Autodesk Inventor part; units mm, degrees
ref_plane "YZ Plane" through (0, 0, 0) normal (1, 0, 0) x (0, 1, 0)
ref_plane "XZ Plane" through (0, 0, 0) normal (0, 1, 0) x (-1, 0, 0)
ref_plane "XY Plane" through (0, 0, 0) normal (0, 0, 1) x (1, 0, 0)
sketch "Sketch2" plane through (0, 0, 0) normal (0, 1, 0) x (-1, 0, 0)
  line L0 (-100, 22.5) -> (100, 22.5)
  line L1 (100, 22.5) -> (100, -22.5)
  line L2 (100, -22.5) -> (-100, -22.5)
  line L3 (-100, -22.5) -> (-100, 22.5)
  line L4 (-100, 22.5) -> (100, -22.5) construction
  line L5 (100, 22.5) -> (-100, -22.5) construction
  line L6 (100, 22.5) -> (95, 22.5)
  line L7 (95, 22.5) -> (95, 27.5)
  line L8 (95, 27.5) -> (100, 27.5)
  line L9 (100, 27.5) -> (100, 22.5)
  line L10 (100, -22.5) -> (95, -22.5)
  line L11 (95, -22.5) -> (95, -27.5)
  line L12 (95, -27.5) -> (100, -27.5)
  line L13 (100, -27.5) -> (100, -22.5)
  line L14 (-100, -22.5) -> (-90, -22.5)
  line L15 (-90, -22.5) -> (-90, -27.5)
  line L16 (-90, -27.5) -> (-100, -27.5)
  line L17 (-100, -27.5) -> (-100, -22.5)
  line L18 (-100, 22.5) -> (-90, 22.5)
  line L19 (-90, 22.5) -> (-90, 27.5)
  line L20 (-90, 27.5) -> (-100, 27.5)
  line L21 (-100, 27.5) -> (-100, 22.5)
  line L22 (94, 17.5) -> (82, 17.5)
  line L23 (82, 17.5) -> (82, 11.5)
  line L24 (82, 11.5) -> (94, 11.5)
  line L25 (94, 11.5) -> (94, 17.5)
  line L26 (70, 17.5) -> (58, 17.5)
  line L27 (70, 11.5) -> (70, 17.5)
  line L28 (58, 11.5) -> (70, 11.5)
  line L29 (58, 17.5) -> (58, 11.5)
  line L30 (46, 17.5) -> (34, 17.5)
  line L31 (46, 11.5) -> (46, 17.5)
  line L32 (34, 11.5) -> (46, 11.5)
  line L33 (34, 17.5) -> (34, 11.5)
  line L34 (22, 17.5) -> (10, 17.5)
  line L35 (22, 11.5) -> (22, 17.5)
  line L36 (10, 11.5) -> (22, 11.5)
  line L37 (10, 17.5) -> (10, 11.5)
  line L38 (-2, 17.5) -> (-14, 17.5)
  line L39 (-2, 11.5) -> (-2, 17.5)
  line L40 (-14, 11.5) -> (-2, 11.5)
  line L41 (-14, 17.5) -> (-14, 11.5)
  line L42 (-26, 17.5) -> (-38, 17.5)
  line L43 (-26, 11.5) -> (-26, 17.5)
  line L44 (-38, 11.5) -> (-26, 11.5)
  line L45 (-38, 17.5) -> (-38, 11.5)
  line L46 (-50, 17.5) -> (-62, 17.5)
  line L47 (-50, 11.5) -> (-50, 17.5)
  line L48 (-62, 11.5) -> (-50, 11.5)
  line L49 (-62, 17.5) -> (-62, 11.5)
  line L50 (-74, 17.5) -> (-86, 17.5)
  line L51 (-74, 11.5) -> (-74, 17.5)
  line L52 (-86, 11.5) -> (-74, 11.5)
  line L53 (-86, 17.5) -> (-86, 11.5)
  line L54 (94, -11.5) -> (82, -11.5)
  line L55 (94, -17.5) -> (94, -11.5)
  line L56 (82, -17.5) -> (94, -17.5)
  line L57 (82, -11.5) -> (82, -17.5)
  line L58 (70, -11.5) -> (58, -11.5)
  line L59 (70, -17.5) -> (70, -11.5)
  line L60 (58, -17.5) -> (70, -17.5)
  line L61 (58, -11.5) -> (58, -17.5)
  line L62 (46, -11.5) -> (34, -11.5)
  line L63 (46, -17.5) -> (46, -11.5)
  line L64 (34, -17.5) -> (46, -17.5)
  line L65 (34, -11.5) -> (34, -17.5)
  line L66 (22, -11.5) -> (10, -11.5)
  line L67 (22, -17.5) -> (22, -11.5)
  line L68 (10, -17.5) -> (22, -17.5)
  line L69 (10, -11.5) -> (10, -17.5)
  line L70 (-2, -11.5) -> (-14, -11.5)
  line L71 (-2, -17.5) -> (-2, -11.5)
  line L72 (-14, -17.5) -> (-2, -17.5)
  line L73 (-14, -11.5) -> (-14, -17.5)
  line L74 (-26, -11.5) -> (-38, -11.5)
  line L75 (-26, -17.5) -> (-26, -11.5)
  line L76 (-38, -17.5) -> (-26, -17.5)
  line L77 (-38, -11.5) -> (-38, -17.5)
  line L78 (-50, -11.5) -> (-62, -11.5)
  line L79 (-50, -17.5) -> (-50, -11.5)
  line L80 (-62, -17.5) -> (-50, -17.5)
  line L81 (-62, -11.5) -> (-62, -17.5)
  line L82 (-74, -11.5) -> (-86, -11.5)
  line L83 (-74, -17.5) -> (-74, -11.5)
  line L84 (-86, -17.5) -> (-74, -17.5)
  line L85 (-86, -11.5) -> (-86, -17.5)
  circle A0 centre (70, 0) radius 2.5
  point P0 (0, 0)
  point P1 (0, 0)
  dimension "d9" = 45
  dimension "d10" = 200
  dimension "d11" = 5
  dimension "d12" = 5
  dimension "d13" = 5
  dimension "d14" = 5
  dimension "d15" = 10
  dimension "d16" = 5
  dimension "d17" = 10
  dimension "d18" = 5
  dimension "d19" = 12
  dimension "d20" = 6
  dimension "d21" = 6
  dimension "d22" = 5
  dimension "d25" = 24
  dimension "d28" = 29
  dimension "d33" = 5
  dimension "d35" = 25
extrude "Extrusion2" add sketch "Sketch2" along normal blind 6
properties part number "phone_holder_slider" material "Acrylic, Clear"
Build history of the part. All positions in model axes, mm. A direction names the side the tool comes from. Give positions to 0.01 mm unless a question says otherwise; leave off trailing zeros. Order: outer loops, then holes, each group sorted by start corner. A loop starts at its lowest first (then second) coordinate and runs counter-clockwise, first axis right, second up. Notation, with made-up numbers: M 25.25,57.5 L 68.25,57.5 A14 cw 68.25,78.5 Z; hole C 43.5,-7.75 d11. An arc over 180 degrees is marked long. Put each result on its own line as item: value.
Item 1: Wall check: probe 1 along Z at (x, y) = (-21, 0.5); probe 2 along X at (y, z) = (5.6, 23); probe 3 along Z at (x, y) = (49.5, 5.15). Give the ranges that are in metal, low to high.
Results are:
probe 1: -22.5 to -17.5, -11.5 to 11.5, 17.5 to 22.5
probe 2: -100 to -95, 90 to 100
probe 3: -22.5 to 22.5
Item 2: Which spindle directions (+Z, -Z, +X, -X, +Y, -Y) get a long thin tool onto all of the face, cutting with end or side? Do faces 3 (the face through (90, 3, 25)), 4 (the face through (90, 3, -25)), 5 (the face through (-40, 3, -11.5)). Say none if no direction does.
Results are:
face 3: +Z, +Y, -Y
face 4: -Z, +Y, -Y
face 5: +Y, -Y
Item 3: Cut at B-B on x = -65. Write the cut outline in (y, z), then the cut area to 3 significant figures.
Results are:
outline: M 0,-22.5 L 6,-22.5 L 6,-17.5 L 0,-17.5 Z; M 0,-11.5 L 6,-11.5 L 6,11.5 L 0,11.5 Z; M 0,17.5 L 6,17.5 L 6,22.5 L 0,22.5 Z
area: 198 mm2
Item 4: Drop flat-ended pins along their axis: pin 1 Ø1.8 at (x, y) = (9.5, 3) entering from -Z; pin 2 Ø1 at (x, y) = (-30.5, 4.5) entering from +Z. Give the stop position or say it passes through.
Results are:
pin 1: z = -22.5
pin 2: z = 22.5
Item 5: Cut at A-A on z = 0. Write the cut outline in (x, y).
Results are:
outline: M -100,0 L -72.5,0 L -72.5,6 L -100,6 Z; M -67.5,0 L 100,0 L 100,6 L -67.5,6 Z
Item 6: Cut at C-C on z = -14.5. Count the separate pieces of the cut face and the enclosed holes in it, then the cut area to 3 significant figures.
Results are:
separate pieces: 9
enclosed holes: 0
area: 624 mm2
Item 7: Pull direction X, two halves, no side cores. Call faces 1 (the face through (-88, 3, -11.5)), 2 (the face through (-100, 3, 0)): +X half, -X half, draft (parallel to the pull), parting line (faces both ways), or undercut.
Results are:
face 1: undercut
face 2: -X half
